Part model, mm, in its own coordinate system. Coordinates: 2 decimals unless noted, no trailing zeros. Loops run counter-clockwise (first coordinate to the right, second up) from the corner with the lowest first, then second, coordinate; pieces in that order, holes last. Notation, with made-up numbers: (-10.5, 66) - (48.5, 66) arc R26 cw to (48.5, 89) - close; hole circle Ø8 at (7.5, 19). An arc over 180 degrees is marked (long way). Use a Markdown table: item, result. Add a question column.
1. Band-saw the part on B-B, the plane z = -3.5. Count the separate pieces of the cut face and the enclosed holes in it, plus the area to 3 significant figures.
2. Pull direction Y, two halves, no side cores. Call faces 1 (the cylindrical face through (33.143, -18.906, -12.522)), 2 (the flat face through (1, 87.277, -13)), 3 (the flat face through (-85.718, 4, -13)): pulls with the +Y half, pulls with the -Y half, needs draft (parallel to the pull), parting line crosses it, or undercut.
3. Wall check: probe 1 along Y at (x, z) = (17.5, -23.5); probe 2 along Y at (x, z) = (58.5, -12.5); probe 3 along X at (y, z) = (5.5, -14). Give the ranges that are in metal, low to high. Write a range as [from, to].
4. Band-saw the part on A-A, the plane y = 11. Give the cut face in (x, z).
from build123d import *

# Parameters (mm, degrees)
F10_W     = 176.685878
F10_H     = 164.152801
F11_DEPTH = 25.4
F7_R      = 9.9
F12_DEPTH = 25.4
F8_R      = 10.5
F13_DEPTH = 25.4
F9_R      = 10.7
F14_DEPTH = 25.4
F0_R      = 7
F15_DEPTH = 25.4
F1_R      = 7.2
F16_DEPTH = 25.4
F3_R      = 7.6
F17_DEPTH = 25.4
F2_R      = 7.4
F18_DEPTH = 25.4
F4_R      = 7.8
F19_DEPTH = 25.4
F5_R      = 8
F5_R_2    = 8.225
F5_R_3    = 8.45
F5_R_4    = 8.65
F20_DEPTH = 25.4
F6_R      = 8.85
F6_R_2    = 9.1
F6_R_3    = 9.3
F6_R_4    = 9.5
F6_R_5    = 9.7
F6_R_6    = 9.9
F6_R_7    = 10.1
F6_R_8    = 10.3
F21_DEPTH = 25.4
F22_R     = 10.9
F23_DEPTH = 25.4
F24_R     = 11.1
F25_DEPTH = 25.4
F26_R     = 11.3
F27_DEPTH = 25.4


with BuildPart() as f11:
    # F10 (on Top) → F11 (new body)
    with BuildSketch(Plane.XY):
        with Locations((2.625104, 5.200521)):
            Rectangle(F10_W, F10_H)
    extrude(amount=-F11_DEPTH)

    # F7 (on Top) → F12 (cut)
    with BuildSketch(Plane.XY):
        with Locations((-56.892078, 61.436351)):
            Circle(F7_R)
    extrude(amount=-F12_DEPTH, mode=Mode.SUBTRACT)

    # F8 (on Top) → F13 (cut)
    with BuildSketch(Plane.XY):
        with Locations((-20.550484, 60.300212)):
            Circle(F8_R)
    extrude(amount=-F13_DEPTH, mode=Mode.SUBTRACT)

    # F9 (on Top) → F14 (cut)
    with BuildSketch(Plane.XY):
        with Locations((12.775544, 62.653594)):
            Circle(F9_R)
    extrude(amount=-F14_DEPTH, mode=Mode.SUBTRACT)

    # F0 (on Top) → F15 (cut)
    with BuildSketch(Plane.XY):
        with Locations((-64.470865, 30.299246)):
            Circle(F0_R)
    extrude(amount=-F15_DEPTH, mode=Mode.SUBTRACT)

    # F1 (on Top) → F16 (cut)
    with BuildSketch(Plane.XY):
        with Locations((-39.056268, 31.34875)):
            Circle(F1_R)
    extrude(amount=-F16_DEPTH, mode=Mode.SUBTRACT)

    # F3 (on Top) → F17 (cut)
    with BuildSketch(Plane.XY):
        with Locations((19.813331, 34.10523)):
            Circle(F3_R)
    extrude(amount=-F17_DEPTH, mode=Mode.SUBTRACT)

    # F2 (on Top) → F18 (cut)
    with BuildSketch(Plane.XY):
        with Locations((-10.968515, 33.251639)):
            Circle(F2_R)
    extrude(amount=-F18_DEPTH, mode=Mode.SUBTRACT)

    # F4 (on Top) → F19 (cut)
    with BuildSketch(Plane.XY):
        with Locations((53.448476, 36.223363)):
            Circle(F4_R)
    extrude(amount=-F19_DEPTH, mode=Mode.SUBTRACT)

    # F5 (on Top) → F20 (cut)
    with BuildSketch(Plane.XY):
        with Locations((-52.422121, 6.954235)):
            Circle(F5_R)
        with Locations((-24.704576, 6.954235)):
            Circle(F5_R_2)
        with Locations((6.08955, 6.954235)):
            Circle(F5_R_3)
        with Locations((41.318376, 4.69443)):
            Circle(F5_R_4)
    extrude(amount=-F20_DEPTH, mode=Mode.SUBTRACT)

    # F6 (on Top) → F21 (cut)
    with BuildSketch(Plane.XY):
        with Locations((-38.879134, -21.031195)):
            Circle(F6_R)
        with Locations((-5.56421, -22.705894)):
            Circle(F6_R_2)
        with Locations((28.14305, -26.74753)):
            Circle(F6_R_3)
        with Locations((62.45793, -28.751563)):
            Circle(F6_R_4)
        with Locations((-61.273046, -48.801046)):
            Circle(F6_R_5)
        with Locations((-24.030989, -53.006683)):
            Circle(F6_R_6)
        with Locations((10.005432, -53.862374)):
            Circle(F6_R_7)
        with Locations((41.005138, -54.6447)):
            Circle(F6_R_8)
    extrude(amount=-F21_DEPTH, mode=Mode.SUBTRACT)

    # F22 (on face) → F23 (cut)
    with BuildSketch(Plane.XY):
        with Locations((38.323849, 57.883684)):
            Circle(F22_R)
    extrude(amount=-F23_DEPTH, mode=Mode.SUBTRACT)

    # F24 (on face) → F25 (cut)
    with BuildSketch(Plane.XY):
        with Locations((65.247305, 56.305163)):
            Circle(F24_R)
    extrude(amount=-F25_DEPTH, mode=Mode.SUBTRACT)

    # F26 (on face) → F27 (cut)
    with BuildSketch(Plane.XY):
        with Locations((67.508779, 3.787257)):
            Circle(F26_R)
    extrude(amount=-F27_DEPTH, mode=Mode.SUBTRACT)


solid = f11.part
Geometry check:
| question | item | result |
|---|---|---|
| 1 | separate pieces | 1 |
| 1 | enclosed holes | 23 |
| 1 | area | 22,800 mm^2 |
| 2 | face 1 | undercut |
| 2 | face 2 | pulls with the +Y half |
| 2 | face 3 | needs draft |
| 3 | probe 1 | y = [-76.88, -60.63], [-47.09, 26.87], [41.34, 53.05], [72.25, 87.28] |
| 3 | probe 2 | y = [-76.88, -37.39], [-20.12, -3.03], [10.61, 30.28], [42.17, 47.49], [65.12, 87.28] |
| 3 | probe 3 | x = [-85.72, -60.29], [-44.56, -32.8], [-16.61, -2.23], [14.41, 32.71], [49.93, 56.34], [78.68, 90.97] |
| 4 | outline | (-85.72, -25.4) - (-59.32, -25.4) - (-59.32, 0) - (-85.72, 0) - close; (-45.52, -25.4) - (-31.87, -25.4) - (-31.87, 0) - (-45.52, 0) - close; (-17.54, -25.4) - (-1.33, -25.4) - (-1.33, 0) - (-17.54, 0) - close; (13.51, -25.4) - (35.4, -25.4) - (35.4, 0) - (13.51, 0) - close; (47.24, -25.4) - (58.81, -25.4) - (58.81, 0) - (47.24, 0) - close; (76.21, -25.4) - (90.97, -25.4) - (90.97, 0) - (76.21, 0) - close |
